The model under review builds one solid part; all positions refer to its coordinate system, in mm. A direction names the side the tool comes from. Coordinates: 2 decimals unless noted, no trailing zeros. Order: outer loops, then holes, each group sorted by start corner. A loop starts at its lowest first (then second) coordinate and runs counter-clockwise, first axis right, second up. Notation, with made-up numbers: (-10, 51.25) -> (5, 51.25) arc R26 ccw to (5, 70.25) -> close; hole circle Ø1 at (-30.75, 17.25). An arc over 180 degrees is marked (long way). Use one line per item in the form item = value.
Autodesk Inventor part; units mm, degrees
ref_plane "YZ Plane" through (0, 0, 0) normal (1, 0, 0) x (0, 1, 0)
ref_plane "XZ Plane" through (0, 0, 0) normal (0, 1, 0) x (-1, 0, 0)
ref_plane "XY Plane" through (0, 0, 0) normal (0, 0, 1) x (1, 0, 0)
sketch "Sketch5" plane through (0, 0, 0) normal (0, 1, 0) x (-1, 0, 0)
  line L0 (-3.1299, 16.302) -> (-3.1299, -27.8812) construction
  line L1 (-3.1299, -27.8812) -> (-19.0358, -27.8812) construction
  line L2 (-19.0358, -27.8812) -> (-19.0358, 16.302) construction
  line L3 (-19.0358, 16.302) -> (-3.1299, 16.302) construction
  line L4 (0, 0) -> (16, 0)
  line L5 (8, 0) -> (8, -24.9508) construction
  line L6 (16, 0) -> (8, -13)
  line L7 (8, -13) -> (0, 0)
  circle A0 centre (8, -15) radius 2.25
  line L8 (0, 0) -> (0, -12.5098) construction
  point P0 (7.8493, -12.7551)
  point P1 (8.1507, -12.7551)
  dimension "d36" = 16
  dimension "d42" = 13
  dimension "d43" = 2
  dimension "d143" = 4.5
extrude "Extrusion4" add sketch "Sketch5" along normal blind 5
sketch "Sketch6" plane through (0, 5, 0) normal (0, 1, 0) x (1, 0, 0)
  arc A0 (-7.8493, 12.7551) -> (-8.1507, 12.7551) centre (-8, 15) ccw
  circle A1 centre (-8, 15) radius 1.75
  line L0 (-16, 0) -> (0, 0)
  line L1 (-16, 0) -> (0, 0) construction
  line L2 (-14.2104, 1) -> (-8, 11.092)
  line L3 (-8.1507, 12.7551) -> (-16, 0)
  line L4 (-8, 11.092) -> (-1.7896, 1)
  line L5 (0, 0) -> (-7.8493, 12.7551)
  line L6 (-14.2104, 1) -> (-1.7896, 1)
  line L7 (-8, 15) -> (-8, 0) construction
  dimension "d46" = 0.5
  dimension "d52" = 1
  dimension "d53" = 1
extrude "Extrusion5" [suppressed]
fillet "Fillet1" radius 1 2 edges at (0, 2.5, 0) (-16, 2.5, 0)
sketch "Sketch9" plane through (0, 0, 0) normal (0, -1, 0) x (1, 0, 0)
  line L0 (-15.5, 3) -> (-0.5, 3)
  line L1 (-0.5, 3) -> (-0.5, -19)
  line L2 (-0.5, -19) -> (-15.5, -19)
  line L3 (-15.5, -19) -> (-15.5, 3)
  line L4 (-15.5, 3) -> (-0.5, -19) construction
  line L5 (-0.5, 3) -> (-15.5, -19) construction
  line L6 (-14.2104, 0) -> (-1.7896, 0)
  line L7 (-8, -15) -> (-8, 0) construction
  arc A0 (-8.1507, -12.7551) -> (-7.8493, -12.7551) centre (-8, -15) ccw construction
  circle A1 centre (-8, -15) radius 2.1568 construction
  point P0 (0, 0)
  point P1 (-8, -8)
  dimension "d75" = 15
  dimension "d76" = 22
  dimension "d77" = 3
extrude "Extrusion7" add sketch "Sketch9" along normal blind 3
sketch "Sketch10" plane through (0, -3, 0) normal (0, -1, 0) x (1, 0, 0)
  line L0 (-0.5, -19) -> (-0.5, 3)
  line L1 (-0.5, -0.75) -> (-1.5, -0.75)
  line L2 (-1.5, -0.75) -> (-1.5, -3.75)
  line L3 (-1.5, -3.75) -> (-0.5, -3.75)
  line L4 (-0.5, -3.75) -> (-0.5, -0.75)
  line L5 (-15.5, 3) -> (-15.5, -19)
  line L6 (-15.5, -0.75) -> (-14.5, -0.75)
  line L7 (-14.5, -0.75) -> (-14.5, -3.75)
  line L8 (-14.5, -3.75) -> (-15.5, -3.75)
  line L9 (-15.5, -3.75) -> (-15.5, -0.75)
  line L10 (-0.5, 3) -> (-15.5, 3)
  point P0 (0, 0)
  point P1 (-15.5, -3.75)
  point P2 (-0.5, -3.75)
  dimension "d80" = 1
  dimension "d81" = 3
  dimension "d82" = 1
  dimension "d83" = 3
  dimension "d84" = 3.75
  dimension "d85" = 3.75
extrude "Extrusion8" add sketch "Sketch10" along normal blind 1.6
sketch "Sketch11" plane through (0, -3, 0) normal (0, -1, 0) x (1, 0, 0)
  line L0 (-9.25, -1.75) -> (-6.75, -1.75)
  line L1 (-6.75, -1.75) -> (-6.75, -3.25)
  line L2 (-6.75, -3.25) -> (-9.25, -3.25)
  line L3 (-9.25, -3.25) -> (-9.25, -1.75)
  line L4 (-8, 0) -> (-8, -15.1696) construction
  line L5 (-15.5, -19) -> (-0.5, -19) construction
  line L6 (-8, -19) -> (-8, 3) construction
  line L7 (-0.5, 3) -> (-15.5, 3) construction
  line L8 (-1.5, -0.75) -> (-1.5, -3.75)
  line L9 (-14.5, -3.75) -> (-14.5, -0.75)
  line L10 (-0.5, -0.75) -> (-1.5, -0.75)
  line L11 (-15.5, -3.75) -> (-15.5, -19)
  line L12 (-6.75, -14.75) -> (-9.25, -14.75)
  line L13 (-9.25, -14.75) -> (-9.25, -16.25)
  line L14 (-9.25, -16.25) -> (-6.75, -16.25)
  line L15 (-6.75, -16.25) -> (-6.75, -14.75)
  line L16 (-6.75, -14.75) -> (-9.25, -16.25) construction
  line L17 (-9.25, -14.75) -> (-6.75, -16.25) construction
  line L18 (-1.5, -3.75) -> (-0.5, -3.75)
  point P0 (0, 0)
  point P1 (-8, -1.75)
  point P2 (-9.25, -2.5)
  point P3 (-8, -3.25)
  point P4 (-8, 0)
  point P5 (-8, -8)
  point P6 (-6.75, -2.5)
  point P7 (-8, -15.5)
  point P8 (-6.75, -15.5)
  dimension "d129" = 7.5
  dimension "d133" = 1.5
  dimension "d136" = 2.5
  dimension "d137" = 1.5
  dimension "d138" = 13
  dimension "d141" = 0.5
extrude "Extrusion9" cut sketch "Sketch11" against normal blind 16
sketch "Sketch13" plane through (0, -3, 0) normal (0, -1, 0) x (1, 0, 0)
  line L0 (-1.5, 2) -> (-14.5, 2)
  line L1 (-14.5, 2) -> (-14.5, -18)
  line L2 (-14.5, -18) -> (-1.5, -18)
  line L3 (-1.5, -18) -> (-1.5, 2)
  line L4 (-0.5, 3) -> (-15.5, 3)
  line L5 (-0.5, -0.75) -> (-0.5, 3)
  line L6 (-15.5, 3) -> (-15.5, -0.75)
  line L7 (-15.5, -19) -> (-0.5, -19)
  point P0 (0, 0)
  point P1 (-15.5, 1.125)
  dimension "d106" = 1
  dimension "d107" = 1
  dimension "d108" = 1
  dimension "d109" = 1
extrude "Extrusion11" cut sketch "Sketch13" against normal blind 2
sketch "Sketch14" plane through (0, -1, 0) normal (0, -1, 0) x (1, 0, 0)
  line L0 (-9.25, -14.75) -> (-9.25, -16.25) construction
  line L1 (-9.25, -15.5) -> (-6.75, -15.5) construction
  line L2 (-6.75, -16.25) -> (-6.75, -14.75) construction
  line L3 (-9.25, -16.25) -> (-6.75, -16.25) construction
  line L4 (-8, -16.25) -> (-8, -1.75) construction
  line L5 (-6.75, -1.75) -> (-9.25, -1.75) construction
  line L6 (-9.25, -1.75) -> (-9.25, -3.25) construction
  line L7 (-9.25, -2.5) -> (-6.75, -2.5) construction
  line L8 (-6.25, -16.25) -> (-9.75, -16.25)
  line L9 (-9.75, -16.25) -> (-9.75, -14.75)
  line L10 (-9.75, -14.75) -> (-6.25, -14.75)
  line L11 (-6.25, -14.75) -> (-6.25, -16.25)
  line L12 (-6.25, -16.25) -> (-9.75, -14.75) construction
  line L13 (-9.75, -16.25) -> (-6.25, -14.75) construction
  line L14 (-6.25, -1.75) -> (-9.75, -1.75)
  line L15 (-9.75, -1.75) -> (-9.75, -3.25)
  line L16 (-9.75, -3.25) -> (-6.25, -3.25)
  line L17 (-6.25, -3.25) -> (-6.25, -1.75)
  line L18 (-6.25, -1.75) -> (-9.75, -3.25) construction
  line L19 (-9.75, -1.75) -> (-6.25, -3.25) construction
  point P0 (0, 0)
  point P1 (-8, -15.5)
  point P2 (-8, -2.5)
  dimension "d139" = 3.5
  dimension "d140" = 1.5
extrude "Extrusion12" cut sketch "Sketch14" against normal blind 1
sketch "Sketch15" plane through (0, -1, 0) normal (0, -1, 0) x (1, 0, 0)
  circle A0 centre (-8, -8.25) radius 1
  line L0 (-8, 0) -> (-8, -15) construction
  circle A1 centre (-8, -8.25) radius 1.7
  line L1 (-14.5, 2) -> (-1.5, 2)
  line L2 (-9.25, -3.25) -> (-6.75, -3.25)
  point P0 (0, 0)
  point P1 (-10.0959, -3.25)
  point P2 (-13.4041, -3.25)
  point P3 (-6.25, -3.25)
  point P4 (-9.75, -3.25)
  dimension "d117" = 2
  dimension "d118" = 0.7
  dimension "d131" = 10.25
extrude "Extrusion13" add sketch "Sketch15" along normal blind 2 contours A0 | A1
sketch "Sketch17" plane through (0, -1, 0) normal (0, -1, 0) x (1, 0, 0)
  point P0 (0, 0)
sketch "Sketch16" plane through (-8, -3, -8.25) normal (0, -1, 0) x (1, 0, 0)
  circle A0 centre (0, 0) radius 1.7
  circle A1 centre (0, 0) radius 1
  point P0 (8, 8.25)
  point P1 (-1.9339, 0.25)
  point P2 (1.9339, 0.25)
  dimension "d123" = 2
  dimension "d60" = 2.5
  dimension "d61" = 0.7
  dimension "d62" = 2.5
  dimension "d63" = 1.5
  dimension "d68" = 13
  dimension "d69" = 3.75
  dimension "d70" = 3.75
  dimension "d72" = 3.75
  dimension "d0" = 15
  dimension "d2" = 10
  dimension "d11" = 5
  dimension "d12" = 1.8
extrude "Extrusion14" cut sketch "Sketch16" against normal blind 5 contours A1
properties part number "NOTGATE"
Item 1: We need section D-D (y = 3.75). Write out the cut boundary in (x, z), plus the area to 3 significant figures.
Results found:
outline = (-15.06, -1.52) -> (-8.15, -12.76) arc R2.25 ccw (long way) to (-7.85, -12.76) -> (-0.94, -1.52) arc R1 ccw to (-1.79, 0) -> (-14.21, 0) arc R1 ccw to start; hole (-9.25, -16.25) -> (-6.75, -16.25) -> (-6.75, -14.75) -> (-9.25, -14.75) -> close; hole (-9.25, -3.25) -> (-6.75, -3.25) -> (-6.75, -1.75) -> (-9.25, -1.75) -> close
area = 111 mm²
Item 2: Draft analysis for pull direction X (two halves, no side actions). For faces 1 (the face through (-8, -1, 3)), 2 (the face through (-9.25, 2, -15)), 3 (the face through (-14.5, -2, -8)), 4 (the face through (-4.442, 2.465, -7.218)), state which applies: released by +X, released by -X, zero draft, split by the parting line, or undercut.
Results found:
face_1 = zero draft
face_2 = undercut
face_3 = undercut
face_4 = released by +X
Item 3: Clearance check with flat-ended pins moving along their axes: pin 1 (2 mm diameter, centred on x = -9, z = -12.5, fed in from -Y); pin 2 (8 mm diameter, centred on x = -12, z = -0.5, fed in from -Y); pin 3 (1.2 mm diameter, centred on y = 3, z = -15, fed in from -X); pin 4 (4 mm diameter, centred on x = -11.5, z = 0.5, fed in from -Y). State where each tip first meets the part, or that it passes through.
Results found:
pin_1 = -1
pin_2 = -4.6
pin_3 = -10.25
pin_4 = -3
Item 4: We need section B-B (y = 1). Write out the cut boundary in (x, z).
Results found:
outline = (-15.06, -1.52) -> (-8.15, -12.76) arc R2.25 ccw (long way) to (-7.85, -12.76) -> (-0.94, -1.52) arc R1 ccw to (-1.79, 0) -> (-14.21, 0) arc R1 ccw to start; hole (-9.25, -16.25) -> (-6.75, -16.25) -> (-6.75, -14.75) -> (-9.25, -14.75) -> close; hole (-9.25, -3.25) -> (-6.75, -3.25) -> (-6.75, -1.75) -> (-9.25, -1.75) -> close; hole circle Ø2 at (-8, -8.25)
Item 5: Tool access review of faces 5 (the face through (-1, -4, -3.75)), 6 (the face through (-11, 0, -10)), 7 (the face through (-8, -2, -18)): name each direction out of +Z, -Z, +X, -X, +Y, -Y from which nothing blocks a thin tool from reaching the whole face with its end or side.
Results found:
face_5 = -Z, +X, -X, -Y
face_6 = +Y
face_7 = -Y
Item 6: To check wall thickness, follow L1, parallel to Z at x = -8, y = -0.6; L2, parallel to Z at x = -8, y = -1.7; L3, parallel to Y at x = -11.5, z = -2. State the ranges of each line that lie inside material, in increasing order. Write a range as from..to.
Results found:
L1 = -19..-16.25, -14.75..-9.25, -7.25..-3.25, -1.75..3
L2 = -19..-18, -9.95..-9.25, -7.25..-6.55, 2..3
L3 = -1..5
Item 7: We need section A-A (y = -1.5). Write out the cut boundary in (x, z), plus the area to 3 significant figures.
Results found:
outline = (-15.5, -19) -> (-0.5, -19) -> (-0.5, 3) -> (-15.5, 3) -> close; circle Ø3.4 at (-8, -8.25); hole (-14.5, -18) -> (-1.5, -18) -> (-1.5, 2) -> (-14.5, 2) -> close; hole circle Ø2 at (-8, -8.25)
area = 75.9 mm²
Item 8: We need section C-C (x = -4). Write out the cut boundary in (y, z).
Results found:
outline = (-3, -19) -> (0, -19) -> (0, -6.5) -> (5, -6.5) -> (5, 0) -> (0, 0) -> (0, 3) -> (-3, 3) -> (-3, 2) -> (-1, 2) -> (-1, -18) -> (-3, -18) -> close
